Part print with two shaded views. Sizes in mm from the minimum x, y, z corner. A direction names the side the tool comes from. Give positions to 0.01 mm unless a question says otherwise; leave off trailing zeros. Write each loop counter-clockwise with the first axis right and the second up, starting at its lowest first coordinate (ties: lowest second). Pieces come first, ordered by that corner, then holes. Notation, with made-up numbers: (55, -39) - (70, -39) arc R22 cw to (70, -5) - close; hole circle Ø11 at (40, 24.5). An arc over 180 degrees is marked (long way). Answer as a JSON object with one key per item and string values.
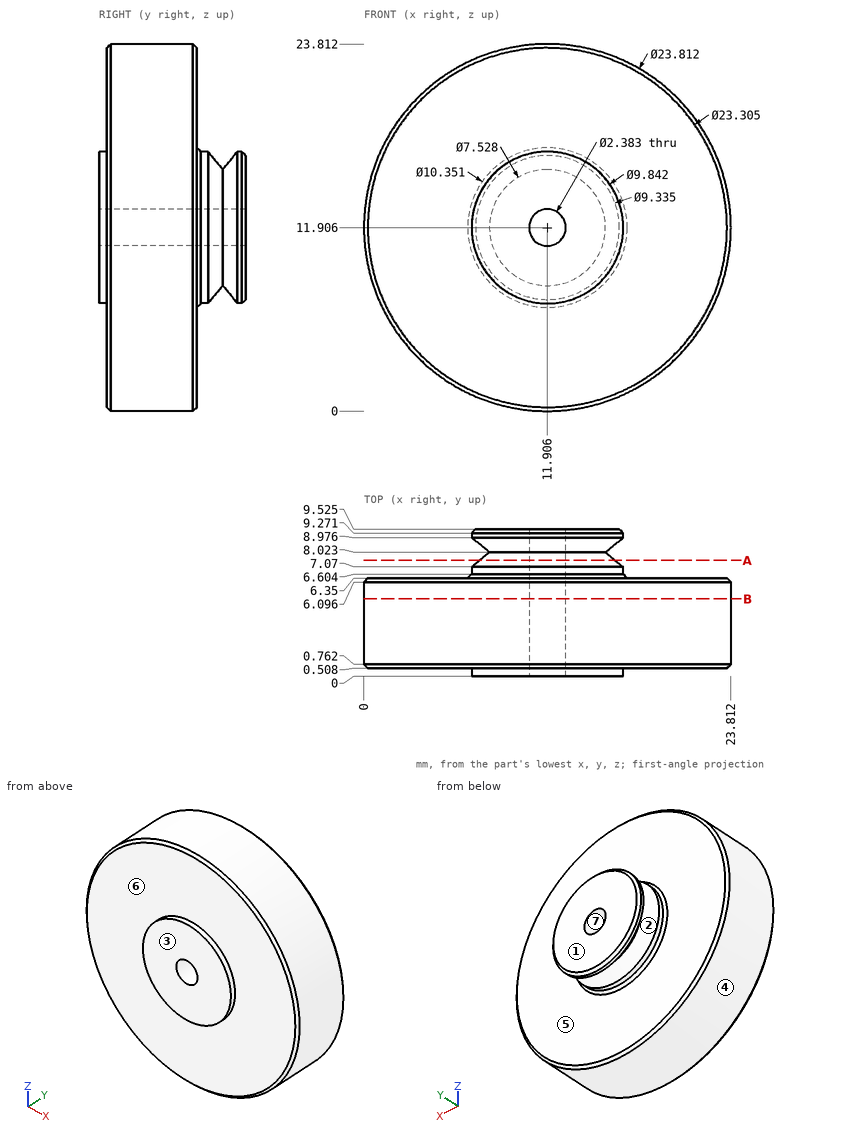
(1) Flat gauge pins, fed straight in: P1, Ø5, axis at x = 9, y = 2, coming from the -Z side; P2, Ø2, axis at y = 6.5, z = 16.5, coming from the -X side; P3, Ø6, axis at x = 20.5, z = 8, coming from the -Y side. Where does each tip first touch, or does it go through?
Answer key:
{"P1": "stops at z = 0.01", "P2": "stops at x = 0.58", "P3": "stops at y = 0.51"}
(2) Saw through at B-B, the plane y = 5. Give the cut face in (x, z).
Answer key:
{"outline": "circle Ø23.81 at (11.91, 11.91); hole circle Ø2.38 at (11.91, 11.91)"}
(3) Saw through at A-A, the plane y = 7.5. Give the cut face in (x, z) (1 decimal).
Answer key:
{"outline": "circle Ø8.8 at (11.9, 11.9); hole circle Ø2.4 at (11.9, 11.9)"}
(4) 3-axis set-ups, long thin cutter, end or side, ignore diameter. For the marked faces 5, 6 and 7: which of +Z, -Z, +X, -X, +Y, -Y reach the whole face in a straight line?
Answer key:
{"face 5": "+Y", "face 6": "-Y", "face 7": "+Y, -Y"}
(5) Pull direction Y, two halves, no side cores. Call the marked faces 1, 2, 3 and 4: pulls with the +Y half, pulls with the -Y half, needs draft (parallel to the pull), parting line crosses it, or undercut.
Answer key:
{"face 1": "pulls with the +Y half", "face 2": "undercut", "face 3": "pulls with the -Y half", "face 4": "needs draft"}
(6) Probe L1, parallel to Y at x = 17.5, z = 6.25; L2, parallel to X at y = 6.25, z = 11.25 (1 decimal); L3, parallel to Z at x = 12.5, y = 1.5 (1 decimal). List the from-to ranges inside material, lowest first. Write a range as [from, to].
Answer key:
{"L1": "y = [0.51, 6.35]", "L2": "x = [0.2, 10.9], [12.9, 23.6]", "L3": "z = [0, 10.9], [12.9, 23.8]"}
